from build123d import *

# Parameters (mm, degrees)
BOSS_EXTRUDE1_DEPTH = 2.5
SKETCH2_R           = 1.2
CUT_EXTRUDE1_DEPTH  = 8
BOSS_EXTRUDE2_START = -25.5
SKETCH6_W           = 4
SKETCH6_H           = 5
BOSS_EXTRUDE2_DEPTH = 18.791796
SKETCH7_W           = 25.4
SKETCH7_H           = 17.5
BOSS_EXTRUDE4_DEPTH = 1.5
FILLET1_R           = 1.5
SKETCH8_R           = 1.2
CUT_EXTRUDE3_DEPTH  = 28


with BuildPart() as part:
    # Sketch1 → Boss-Extrude1 (new body, symmetric)
    with BuildSketch(Plane.XY):
        with BuildLine():
            Line((5.5, 0), (12.7, 0))
            Line((12.7, 0), (12.7, -1.5))
            Line((12.7, -1.5), (6.837397166, -1.5))
            ThreePointArc((6.837397166, -1.5), (0, -7), (-6.837397166, -1.5))
            Line((-6.837397166, -1.5), (-12.7, -1.5))
            Line((-12.7, -1.5), (-12.7, 0))
            Line((-12.7, 0), (-5.5, 0))
            ThreePointArc((-5.5, 0), (0, -5.5), (5.5, 0))
        make_face()
    extrude(amount=BOSS_EXTRUDE1_DEPTH, both=True)

    # Sketch2 → Cut-Extrude1 (cut, through all)
    with BuildSketch(Plane(origin=(0, 0, 0), x_dir=(1, 0, 0), z_dir=(0, 1, 0))):
        with Locations((-10.2, 0)):
            Circle(SKETCH2_R)
        with Locations((10.2, 0)):
            Circle(SKETCH2_R)
    extrude(amount=-CUT_EXTRUDE1_DEPTH, mode=Mode.SUBTRACT)

    # Sketch6 → Boss-Extrude2 (add)
    with BuildSketch(Plane(origin=(0, 0, 0), x_dir=(1, 0, 0), z_dir=(0, 1, 0)).offset(BOSS_EXTRUDE2_START)):
        Rectangle(SKETCH6_W, SKETCH6_H)
    extrude(amount=BOSS_EXTRUDE2_DEPTH)

    # Sketch7 → Boss-Extrude4 (add)
    with BuildSketch(Plane.XZ.offset(25.5)):
        with Locations((0, 6.25)):
            Rectangle(SKETCH7_W, SKETCH7_H)
    extrude(amount=BOSS_EXTRUDE4_DEPTH)

    # Fillet1
    fillet1_edges = [part.edges().sort_by_distance(p)[0] for p in [
        (6.837397166, -1.5, 0),
        (-6.837397166, -1.5, 0),
        (-2, -25.5, 0),
        (0, -25.5, 2.5),
        (2, -25.5, 0),
        (-2, -6.708204, 0),
        (2, -6.708204, 0),
    ]]
    fillet(fillet1_edges, radius=FILLET1_R)

    # Sketch8 → Cut-Extrude3 (cut, through all)
    with BuildSketch(Plane(origin=(0, 0, 0), x_dir=(1, 0, 0), z_dir=(0, 1, 0))):
        with Locations((-5, -12.5)):
            Circle(SKETCH8_R)
        with Locations((5, -12.5)):
            Circle(SKETCH8_R)
    extrude(amount=-CUT_EXTRUDE3_DEPTH, mode=Mode.SUBTRACT)


solid = part.part
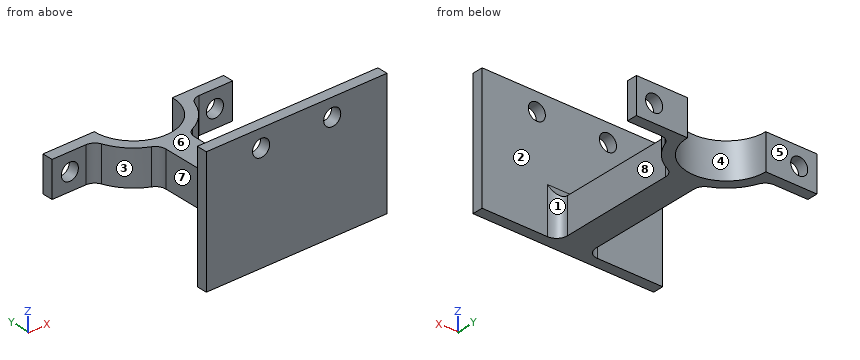
Could you check a few things on this model? Use its own coordinates, in mm. Face numbers are marked on the shaded views. A direction names the side the tool comes from. Give positions to 0.01 mm unless a question says otherwise; leave off trailing zeros. Write each loop counter-clockwise with the first axis right and the second up, starting at its lowest first coordinate (ties: lowest second). Pieces come first, ordered by that corner, then holes. Notation, with made-up numbers: (13, -16) -> (55, -16) arc R25 cw to (55, 7) -> close; hole circle Ø7 at (50.5, -16.5). An arc over 180 degrees is marked (long way). Answer as CSV lines item,"result". Start each with the question number.
(1) Please list where these lines run through material, in increasing order: line 1 (X direction, y = -25.9, z = 12.5); line 2 (Z direction, x = -5, y = -26.6); line 3 (Y direction, x = -1, z = 12.25).
(2) If we mould it in two halves opening along Y, with no side actions, what happens to the marked faces 5, 6, 7 and 8? For each: +Y half, -Y half, draft (parallel to the pull), parting line (faces both ways), or undercut.
(3) Which directions (+Z, -Z, +X, -X, +Y, -Y) give clear straight access to the entire face, cutting with the end or side of a thin tool? Please do the marked faces 1, 2, 3 and 4.
(4) I'm going to push flat-ended pins straight in: pin 1 Ø4 at (x, z) = (-5, 12.5) entering from +Y; pin 2 Ø2 at (x, z) = (-9, 0.5) entering from +Y; pin 3 Ø1.5 at (y, z) = (-16.5, 1) entering from -X; pin 4 Ø7 at (x, y) = (2, -11) entering from +Z. Where does each tip first touch, or does it pass through?
(5) If we section it at A-A, the plane z = 12.5: Write out the boundary of the cut face in (x, y), and give its area (3 significant figures).
(6) If we section it at B-B, the plane x = -10.2: Write out the boundary of the cut face in (y, z), and give its area (4 significant figures).
(7) If we section it at D-D, the plane z = 0: Give the number of separate pieces and of enclosed holes in the cut face, and give its area (3 significant figures).
(8) If we section it at C-C, the plane x = 0: Write out the boundary of the cut face in (y, z).
Answer list:
1,line 1,"-12.7 to -6.2, -3.8 to 3.8, 6.2 to 12.7"
1,line 2,"-2.5 to 11.3, 13.7 to 15"
1,line 3,"-27 to -25.5"
2,face 5,"+Y half"
2,face 6,"draft"
2,face 7,"undercut"
2,face 8,"undercut"
3,face 1,"+Z, -Z, +X"
3,face 2,"+Z"
3,face 3,"+Z, -Z, -X"
3,face 4,"+Z, -Z, +Y"
4,pin 1,"y = -25.5"
4,pin 2,"y = 0"
4,pin 3,"x = -2"
4,pin 4,"z = 2.5"
5,outline,"(-12.7, -27) -> (-6.2, -27) -> (-6.2, -25.5) -> (-12.7, -25.5) -> close; (-3.8, -27) -> (3.8, -27) -> (3.8, -25.5) -> (-3.8, -25.5) -> close; (6.2, -27) -> (12.7, -27) -> (12.7, -25.5) -> (6.2, -25.5) -> close"
5,area,"30.9 mm^2"
6,outline,"(-27, -2.5) -> (-25.5, -2.5) -> (-25.5, 15) -> (-27, 15) -> close; (-1.5, -2.5) -> (0, -2.5) -> (0, -1.2) -> (-1.5, -1.2) -> close; (-1.5, 1.2) -> (0, 1.2) -> (0, 2.5) -> (-1.5, 2.5) -> close"
6,area,"30.15 mm^2"
7,separate pieces,"3"
7,enclosed holes,"0"
7,area,"154 mm^2"
8,outline,"(-27, -2.5) -> (-5.5, -2.5) -> (-5.5, 2.5) -> (-24, 2.5) arc R1.5 cw to (-25.5, 4) -> (-25.5, 15) -> (-27, 15) -> close"
